CAD build for the part. Positions are in the model's coordinates, mm. Round coordinates to 2 decimals unless told otherwise and drop trailing zeros. Loops run counter-clockwise (first coordinate to the right, second up) from the corner with the lowest first, then second, coordinate; pieces in that order, holes last.
```python
from build123d import *

# Parameters (mm, degrees)
AUFSATZ_LINEAR_AUSTRAGEN1_DEPTH = 12
M10_GEWINDEBOHRUNG1_D           = 8.5
M10_GEWINDEBOHRUNG1_DEPTH       = 37.5
M10_GEWINDEBOHRUNG1_TIP         = 2.553657631
M10_GEWINDEBOHRUNG2_D           = 8.5
M10_GEWINDEBOHRUNG2_DEPTH       = 37.5
M10_GEWINDEBOHRUNG2_TIP         = 2.553657631
VERRUNDUNG1_R                   = 10


with BuildPart() as part:
    # Skizze1 → Aufsatz-Linear austragen1 (new body)
    with BuildSketch(Plane.XY):
        Polygon((100, 0), (100, 100), (0, 50), (0, 0), align=None)
    extrude(amount=AUFSATZ_LINEAR_AUSTRAGEN1_DEPTH)

    # M10 Gewindebohrung1
    with Locations(Plane(origin=(0, 0, 0), x_dir=(-1, 0, 0), z_dir=(0, -1, 0))):
        with Locations((-15, -6), (-85, -6)):
            Hole(M10_GEWINDEBOHRUNG1_D / 2, depth=M10_GEWINDEBOHRUNG1_DEPTH)
            with Locations((0, 0, -(M10_GEWINDEBOHRUNG1_DEPTH + M10_GEWINDEBOHRUNG1_TIP / 2))):  # 118° drill point
                Cone(0, M10_GEWINDEBOHRUNG1_D / 2, M10_GEWINDEBOHRUNG1_TIP, mode=Mode.SUBTRACT)

    # M10 Gewindebohrung2
    with Locations(Plane(origin=(100, 0, 0), x_dir=(0, 0, -1), z_dir=(1, 0, 0))):
        with Locations((-6, 50), (-6, 80)):
            Hole(M10_GEWINDEBOHRUNG2_D / 2, depth=M10_GEWINDEBOHRUNG2_DEPTH)
            with Locations((0, 0, -(M10_GEWINDEBOHRUNG2_DEPTH + M10_GEWINDEBOHRUNG2_TIP / 2))):  # 118° drill point
                Cone(0, M10_GEWINDEBOHRUNG2_D / 2, M10_GEWINDEBOHRUNG2_TIP, mode=Mode.SUBTRACT)

    # Verrundung1
    verrundung1_edges = [part.edges().sort_by_distance(p)[0] for p in [
        (0, 50, 6),
    ]]
    fillet(verrundung1_edges, radius=VERRUNDUNG1_R)


solid = part.part
```
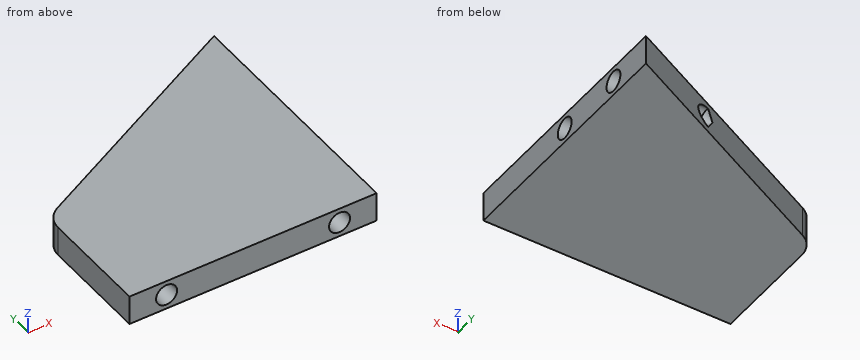
Item 1: Cut at A-A, the plane x = 90.5. Give the cut face in (y, z).
Answers follow:
outline: (0, 0) - (95.25, 0) - (95.25, 12) - (0, 12) - close; hole circle Ø8.5 at (50, 6); hole circle Ø8.5 at (80, 6)
Item 2: Flat gauge pins, fed straight in: P1, Ø1, axis at x = 62, z = 1.5, coming from the -Y side; P2, Ø6, axis at y = 84, z = 10.5, coming from the -X side; P3, Ø5, axis at x = 85, z = 6, coming from the -Y side; P4, Ø2, axis at x = 77, z = 7.5, coming from the +Y side. Where does each tip first touch, or does it go through?
Answers follow:
P1: stops at y = 0
P2: stops at x = 62
P3: stops at y = 38.55
P4: stops at y = 89
Item 3: Cut at B-B, the plane y = 30.5. Give the cut face in (x, z), plus the area to 3 significant figures.
Answers follow:
outline: (0, 0) - (100, 0) - (100, 12) - (0, 12) - close; hole circle Ø8.5 at (15, 6); hole circle Ø8.5 at (85, 6)
area: 1,090 mm2
Item 4: Probe line 1 (Y direction, x = 91, z = 3.75); line 2 (Y direction, x = 92.5, z = 6); line 3 (X direction, y = 25, z = 9.75). List the from-to ranges inside material, lowest first.
Answers follow:
line 1: y = 0 to 46.39, 53.61 to 76.39, 83.61 to 95.5
line 2: y = 0 to 45.75, 54.25 to 75.75, 84.25 to 96.25
line 3: x = 0 to 13, 17 to 83, 87 to 100
Item 5: Cut at C-C, the plane y = 59. Give the cut face in (x, z), plus the area to 3 significant figures.
Answers follow:
outline: (18, 0) - (100, 0) - (100, 12) - (18, 12) - close
area: 984 mm2
